Check sheet for the modelled part. Datum: model origin and axes. Units: mm. A direction names the side the tool comes from. Coordinates: 2 decimals unless noted, no trailing zeros. Loops run counter-clockwise (first coordinate to the right, second up) from the corner with the lowest first, then second, coordinate; pieces in that order, holes last. Notation, with made-up numbers: (80, -16) - (126, -16) arc R13 ccw to (126, -10) - close; hole circle Ø10 at (33.5, 63). An arc over 180 degrees is marked (long way). Write each question's results on one line, items separated by ' | '. Start each with the question number.
1. Cross-section at C-C (x = 3). Record the cut outline in (y, z), and give its area (3 significant figures).
2. Draft check along Y on faces 3 (the face through (-17.595, 6, -4)), 4 (the face through (22.601, 36.884, -3.698)), 5 (the face through (-15.79, -23.694, -3.698)), 6 (the face through (18.605, -15, -4)). Enter one of: released by +Y, released by -Y, zero draft, split by the parting line, or undercut.
3. Thickness scan on line 1 (Y direction, x = -12, z = -2.5); line 2 (X direction, y = -16, z = -6.75); line 3 (X direction, y = 17, z = -5.25). Record the ranges inside material, lowest first. Write a range as [from, to].
4. Cross-section at D-D (z = -4.25). Record the cut outline in (x, y).
5. Gauge pin test, flat end, axial feed: P1, Ø2.5, axis at x = -12.09, y = 33.09, coming from the +Z side. Record the tip position at first contact, or that the pin passes through.
6. Tool access check on faces 1 (the face through (15.948, -20.005, -3.698)), 2 (the face through (4, 0, -7.5)). Record the directions out of +Z, -Z, +X, -X, +Y, -Y that give a thin tool (end or side, any length) a straight path to the whole face; none if there is none.
7. Cross-section at B-B (x = 15). Record the cut outline in (y, z), and give its area (3 significant figures).
8. Cross-section at A-A (y = 28). Record the cut outline in (x, z), and give its area (3 significant figures).
```python
from build123d import *

# Parameters (mm, degrees)
SKETCH_1_R      = 12.5
SKETCH_1_R_2    = 1.6
EXTRUDE_1_DEPTH = 7.5


with BuildPart() as part:
    # 草图1 → 凸台-拉伸1 (new body)
    with BuildSketch(Plane.XY):
        with BuildLine():
            Line((-11.594594595, 38.594594595), (18.405405405, 38.594594595))
            ThreePointArc((18.405405405, 38.594594595), (22.648046093, 36.837235282), (24.405405405, 32.594594595))
            Line((24.405405405, 32.594594595), (24.405405405, -19.405405405))
            ThreePointArc((24.405405405, -19.405405405), (22.648046093, -23.648046093), (18.405405405, -25.405405405))
            Line((18.405405405, -25.405405405), (-11.594594595, -25.405405405))
            ThreePointArc((-11.594594595, -25.405405405), (-15.837235282, -23.648046093), (-17.594594595, -19.405405405))
            Line((-17.594594595, -19.405405405), (-17.594594595, 32.594594595))
            ThreePointArc((-17.594594595, 32.594594595), (-15.837235282, 36.837235282), (-11.594594595, 38.594594595))
        make_face()
        with Locations((3.405405405, 17.594594595)):
            Circle(SKETCH_1_R, mode=Mode.SUBTRACT)
        with Locations((-12.094594595, 33.094594595)):
            Circle(SKETCH_1_R_2, mode=Mode.SUBTRACT)
        with Locations((18.905405405, 33.094594595)):
            Circle(SKETCH_1_R_2, mode=Mode.SUBTRACT)
        with Locations((18.905405405, 2.094594595)):
            Circle(SKETCH_1_R_2, mode=Mode.SUBTRACT)
        with Locations((-12.094594595, 2.094594595)):
            Circle(SKETCH_1_R_2, mode=Mode.SUBTRACT)
        with BuildLine():
            Line((13.405405405, -12.605405405), (13.405405405, -17.40540541))
            ThreePointArc((13.405405405, -17.40540541), (16.005405405, -20.00540541), (18.605405405, -17.40540541))
            Line((18.605405405, -17.40540541), (18.605405405, -12.605405405))
            ThreePointArc((18.605405405, -12.605405405), (16.005405405, -10.005405405), (13.405405405, -12.605405405))
        make_face(mode=Mode.SUBTRACT)
        with BuildLine():
            Line((-11.594594595, -12.605405405), (-11.594594595, -17.40540541))
            ThreePointArc((-11.594594595, -17.40540541), (-8.994594595, -20.00540541), (-6.394594595, -17.40540541))
            Line((-6.394594595, -17.40540541), (-6.394594595, -12.605405405))
            ThreePointArc((-6.394594595, -12.605405405), (-8.994594595, -10.005405405), (-11.594594595, -12.605405405))
        make_face(mode=Mode.SUBTRACT)
    extrude(amount=-EXTRUDE_1_DEPTH)


solid = part.part
```
Established:
1) outline: (-25.41, -7.5) - (5.1, -7.5) - (5.1, 0) - (-25.41, 0) - close; (30.09, -7.5) - (38.59, -7.5) - (38.59, 0) - (30.09, 0) - close | area: 293 mm^2
2) face 3: zero draft | face 4: released by +Y | face 5: released by -Y | face 6: undercut
3) line 1: [-25.39, 0.5], [3.69, 31.5], [34.69, 38.58] | line 2: [-17.59, -11.59], [-6.39, 13.41], [18.61, 24.41] | line 3: [-17.59, -9.08], [15.89, 24.41]
4) outline: (-17.59, -19.41) arc R6 ccw to (-11.59, -25.41) - (18.41, -25.41) arc R6 ccw to (24.41, -19.41) - (24.41, 32.59) arc R6 ccw to (18.41, 38.59) - (-11.59, 38.59) arc R6 ccw to (-17.59, 32.59) - close; hole circle Ø3.2 at (-12.09, 2.09); hole circle Ø3.2 at (-12.09, 33.09); hole (-11.59, -17.41) arc R2.6 ccw to (-6.39, -17.41) - (-6.39, -12.61) arc R2.6 ccw to (-11.59, -12.61) - close; hole circle Ø25 at (3.41, 17.59); hole (13.41, -17.41) arc R2.6 ccw to (18.61, -17.41) - (18.61, -12.61) arc R2.6 ccw to (13.41, -12.61) - close; hole circle Ø3.2 at (18.91, 2.09); hole circle Ø3.2 at (18.91, 33.09)
5) P1: through
6) face 1: +Z, -Z | face 2: -Z, +X, -X, +Y, -Y
7) outline: (-25.41, -7.5) - (-19.8, -7.5) - (-19.8, 0) - (-25.41, 0) - close; (-10.21, -7.5) - (12.92, -7.5) - (12.92, 0) - (-10.21, 0) - close; (22.27, -7.5) - (38.59, -7.5) - (38.59, 0) - (22.27, 0) - close | area: 338 mm^2
8) outline: (-17.59, -7.5) - (-3.52, -7.5) - (-3.52, 0) - (-17.59, 0) - close; (10.33, -7.5) - (24.41, -7.5) - (24.41, 0) - (10.33, 0) - close | area: 211 mm^2
